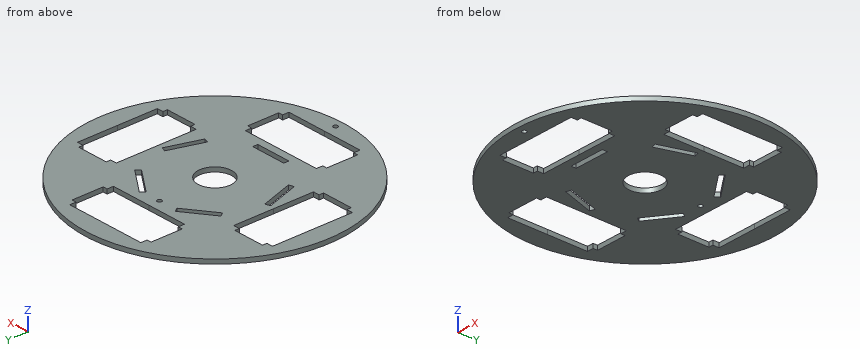
from build123d import *

# Parameters (mm, degrees)
MODEL_R             = 147.220888612
MODEL_R_2           = 2.54
MODEL_R_3           = 19.05
MODEL_W             = 40.000341048
MODEL_H             = 5.842
BOSS_EXTRUDE1_DEPTH = 5.0038


with BuildPart() as part:
    # Model → Boss-Extrude1 (new body)
    with BuildSketch(Plane.XY):
        with Locations((150.608180965, -149.916372011)):
            Circle(MODEL_R)
        with Locations((150.608180965, -288.178437552)):
            Circle(MODEL_R_2, mode=Mode.SUBTRACT)
        with Locations((150.608180965, -149.916372011)):
            Circle(MODEL_R_3, mode=Mode.SUBTRACT)
        with Locations((150.608395424, -86.435544776)):
            Circle(MODEL_R_2, mode=Mode.SUBTRACT)
        Polygon((75.097257942, -195.636586469), (75.097257942, -149.916586488), (75.097650189, -104.19658647), (67.880551818, -104.196555511), (67.880573609, -99.116555511), (32.320573609, -99.116402971), (32.320551818, -104.196402971), (25.103453446, -104.196372012), (25.103453446, -149.916371999), (25.103061199, -195.636372011), (32.32015957, -195.63640297), (32.320137779, -200.71640297), (67.880137779, -200.71655551), (67.88015957, -195.63655551), align=None, mode=Mode.SUBTRACT)
        with Locations((150.651713387, -213.962635212)):
            Rectangle(MODEL_W, MODEL_H, mode=Mode.SUBTRACT)
        Polygon((93.11237376, -189.673088704), (80.751588595, -151.630503696), (86.307660763, -149.825226415), (98.668445928, -187.867811423), align=None, mode=Mode.SUBTRACT)
        Polygon((95.030114956, -107.520111007), (127.391070645, -84.008500452), (130.824912089, -88.734777734), (98.4639564, -112.246388288), align=None, mode=Mode.SUBTRACT)
        Polygon((196.328395424, -225.427295034), (150.608395424, -225.427295034), (104.888395425, -225.426902787), (104.888364466, -232.644001159), (99.808364466, -232.643979367), (99.808211925, -268.203979367), (104.888211925, -268.204001158), (104.888180966, -275.42109953), (150.608180967, -275.42109953), (196.328180965, -275.421491778), (196.328211924, -268.204393406), (201.408211924, -268.204415197), (201.408364465, -232.644415198), (196.328364465, -232.644393406), align=None, mode=Mode.SUBTRACT)
        Polygon((104.887966507, -74.405448987), (150.607966472, -74.405448987), (196.327966506, -74.405841235), (196.327997465, -67.188742863), (201.407997465, -67.188764655), (201.408150006, -31.628764655), (196.328150006, -31.628742863), (196.328180965, -24.411644492), (150.608181003, -24.411644492), (104.888180965, -24.411252244), (104.888150006, -31.628350616), (99.808150007, -31.628328824), (99.807997466, -67.188328824), (104.887997466, -67.188350615), align=None, mode=Mode.SUBTRACT)
        Polygon((226.119103989, -104.196157552), (226.119103989, -149.916157498), (226.118711741, -195.636157551), (233.335810113, -195.63618851), (233.335788322, -200.71618851), (268.895788321, -200.716341051), (268.895810113, -195.636341051), (276.112908485, -195.63637201), (276.112908485, -149.916372061), (276.113300732, -104.196372011), (268.89620236, -104.196341052), (268.896224152, -99.116341052), (233.336224152, -99.116188511), (233.336202361, -104.196188511), align=None, mode=Mode.SUBTRACT)
        Polygon((173.754854348, -83.957325021), (206.115810037, -107.468935576), (202.681968593, -112.195212857), (170.321012904, -88.683602302), align=None, mode=Mode.SUBTRACT)
        Polygon((220.491677852, -151.547700109), (208.130892687, -189.590285117), (202.574820519, -187.785007836), (214.935605684, -149.742422828), align=None, mode=Mode.SUBTRACT)
    extrude(amount=BOSS_EXTRUDE1_DEPTH)


solid = part.part
Work out the finished part from the listing and answer in its coordinate system (mm). Give positions to 0.01 mm unless a question says otherwise; leave off trailing zeros. Write each loop counter-clockwise with the first axis right and the second up, starting at its lowest first coordinate (ties: lowest second). Pieces come first, ordered by that corner, then holes.
Q1. Straight lines are drawn through the part: L1, parallel to Y at x = 196, z = 2.35; L2, parallel to X at y = -186.5, z = 3.2; L3, parallel to Y at x = 145.5, z = 3.8. For each, find the intervals that lie inside material, in ascending order.
Answer:
L1: y = -289.96 to -275.42, -225.43 to -107.34, -100.12 to -74.41, -24.41 to -9.87
L2: x = 8.01 to 25.1, 75.1 to 92.08, 98.22 to 202.99, 209.13 to 226.12, 276.11 to 293.21
L3: y = -297.05 to -275.42, -225.43 to -216.88, -211.04 to -168.27, -131.56 to -74.41, -24.41 to -2.78
Q2. The part is cut by section D-D on y = -59.5. Give the vertices of the cut face in (x, z), and give its area (3 significant figures).
Answer:
outline: (34.42, 0) - (99.81, 0) - (99.81, 5) - (34.42, 5) - close; (201.41, 0) - (266.79, 0) - (266.79, 5) - (201.41, 5) - close
area: 654 mm2
Q3. The part is cut by section A-A on y = -164. Give the vertices of the cut face in (x, z), and give its area (3 significant figures).
Answer:
outline: (4.06, 0) - (25.1, 0) - (25.1, 5) - (4.06, 5) - close; (75.1, 0) - (84.77, 0) - (84.77, 5) - (75.1, 5) - close; (90.91, 0) - (137.78, 0) - (137.78, 5) - (90.91, 5) - close; (163.44, 0) - (210.3, 0) - (210.3, 5) - (163.44, 5) - close; (216.45, 0) - (226.12, 0) - (226.12, 5) - (216.45, 5) - close; (276.11, 0) - (297.15, 0) - (297.15, 5) - (276.11, 5) - close
area: 776 mm2
Q4. The part is cut by section B-B on x = 45. Give the vertices of the cut face in (y, z), and give its area (3 significant figures).
Answer:
outline: (-252.49, 0) - (-200.72, 0) - (-200.72, 5) - (-252.49, 5) - close; (-99.12, 0) - (-47.34, 0) - (-47.34, 5) - (-99.12, 5) - close
area: 518 mm2
Q5. Given pin 1 (3 mm diameter, centred on x = 49, z = 4.5, fed in from +Y); pin 2 (4 mm diameter, centred on x = 150.61, y = -288.18, fed in from +Z); pin 3 (3 mm diameter, centred on y = -229, z = 1.5, fed in from -X); pin 4 (1.5 mm diameter, centred on x = 200, z = 3, fed in from -Y), each flat-ended and moving along its own axis, determine where each tip first touches the part or whether it passes through.
Answer:
pin 1: stops at y = -41.97
pin 2: passes through
pin 3: stops at x = 25.49
pin 4: stops at y = -288.87
Q6. The part is cut by section C-C on y = -126. Give the vertices of the cut face in (x, z), and give its area (3 significant figures).
Answer:
outline: (5.34, 0) - (25.1, 0) - (25.1, 5) - (5.34, 5) - close; (75.1, 0) - (226.12, 0) - (226.12, 5) - (75.1, 5) - close; (276.11, 0) - (295.87, 0) - (295.87, 5) - (276.11, 5) - close
area: 953 mm2
